Source: CAD feature listing. Evaluate the final solid. Frame: model axes, mm. A direction names the side the tool comes from. Give positions to 0.01 mm unless a question says otherwise; leave off trailing zeros. Order: outer loops, then holes, each group sorted by start corner. A loop starts at its lowest first (then second) coordinate and runs counter-clockwise, first axis right, second up. Notation, with made-up numbers: (60.25, 37.25) - (102.25, 37.25) arc R21 cw to (102.25, 46.25) - close; hole circle Ø9 at (27, 56). An arc over 180 degrees is marked (long way). Use CSV: the item, a comma, the result in double quotes.
```python
from build123d import *

# Parameters (mm, degrees)
F0_R     = 3.9142983579
F0_R_2   = 3.3882320549
F0_R_3   = 3.3768548991
F1_DEPTH = 2
F0_R_4   = 8.4535282778
F0_R_5   = 8.4613165319
F5_DEPTH = 6
F6_DEPTH = 6
F7_DEPTH = 6.096


# Not quite as in the source:
# - the program builds the solid bodies; features that only make, move or delete a surface that nothing else refers to are left out


with BuildPart() as f1:
    # F0 (on Top) → F1 (new body)
    with BuildSketch(Plane.XY):
        with BuildLine():
            Line((-5.016844254, 60.8599856496), (-5.016844254, 55.3855970502))
            Line((-5.016844254, 55.3855970502), (27.1643232554, 55.3855970502))
            Line((27.1643232554, 55.3855970502), (27.1643232554, 72.5930482149))
            ThreePointArc((27.1643232554, 72.5930482149), (15.3743446714, 74.0537278173), (9.8619121261, 84.5775231091))
            ThreePointArc((9.8619121261, 84.5775231091), (-38.0783668351, 114.5002429814), (-86.734496244, 85.7561899899))
            ThreePointArc((-86.734496244, 85.7561899899), (-89.789886214, 77.2334083533), (-97.5642204285, 72.5930482149))
            Line((-97.5642204285, 72.5930482149), (-97.5642204285, 55.3855970502))
            Line((-97.5642204285, 55.3855970502), (-82.5288370252, 55.3855970502))
            Line((-82.5288370252, 55.3855970502), (-62.9575885832, 55.3855970502))
            Line((-62.9575885832, 55.3855970502), (-62.9575885832, 60.8599856496))
            ThreePointArc((-62.9575885832, 60.8599856496), (-33.9872164186, 89.8303578142), (-5.016844254, 60.8599856496))
        make_face()
        with Locations((-86.9268402457, 61.0230416059)):
            Circle(F0_R, mode=Mode.SUBTRACT)
        with Locations((-72.1179321408, 60.8599856496)):
            Circle(F0_R, mode=Mode.SUBTRACT)
        with Locations((-68.8042789698, 85.551418364)):
            Circle(F0_R_2, mode=Mode.SUBTRACT)
        with Locations((4.3670018204, 60.8045533299)):
            Circle(F0_R, mode=Mode.SUBTRACT)
        with Locations((19.1759099253, 60.7153773308)):
            Circle(F0_R, mode=Mode.SUBTRACT)
        with Locations((-0.4634411598, 85.6597200036)):
            Circle(F0_R_3, mode=Mode.SUBTRACT)
        with Locations((-56.8258166313, 96.0706025362)):
            Circle(F0_R_3, mode=Mode.SUBTRACT)
        with Locations((-42.8707525134, 101.2179628015)):
            Circle(F0_R_3, mode=Mode.SUBTRACT)
        with Locations((-11.1492751166, 95.5843403935)):
            Circle(F0_R_3, mode=Mode.SUBTRACT)
        with Locations((-24.9121841043, 101.1035814881)):
            Circle(F0_R_3, mode=Mode.SUBTRACT)
    extrude(amount=F1_DEPTH)

    # F0 (on Top) → F5 (join)
    with BuildSketch(Plane.XY):
        with BuildLine():
            ThreePointArc((30.7714908133, 66.0106175583), (42.611434574, 81.0345848644), (36.6692617536, 99.2168411613))
            ThreePointArc((36.6692617536, 99.2168411613), (-37.7049289316, 128.8806796099), (-111.8238263521, 98.5845974088))
            ThreePointArc((-111.8238263521, 98.5845974088), (-116.4247817384, 79.7587957054), (-100.7084514224, 68.4196351703))
            Line((-100.7084514224, 68.4196351703), (-100.7084514224, 49.9112084508))
            Line((-100.7084514224, 49.9112084508), (-62.9575885832, 49.9112084508))
            Line((-62.9575885832, 49.9112084508), (-62.9575885832, 55.3855970502))
            Line((-62.9575885832, 55.3855970502), (-82.5288370252, 55.3855970502))
            Line((-82.5288370252, 55.3855970502), (-97.5642204285, 55.3855970502))
            Line((-97.5642204285, 55.3855970502), (-97.5642204285, 72.5930482149))
            ThreePointArc((-97.5642204285, 72.5930482149), (-89.789886214, 77.2334083533), (-86.734496244, 85.7561899899))
            ThreePointArc((-86.734496244, 85.7561899899), (-38.0783668351, 114.5002429814), (9.8619121261, 84.5775231091))
            ThreePointArc((9.8619121261, 84.5775231091), (15.3743446714, 74.0537278173), (27.1643232554, 72.5930482149))
            Line((27.1643232554, 72.5930482149), (27.1643232554, 55.3855970502))
            Line((27.1643232554, 55.3855970502), (-5.016844254, 55.3855970502))
            Line((-5.016844254, 55.3855970502), (-5.016844254, 49.9112084508))
            Line((-5.016844254, 49.9112084508), (30.7714908133, 49.9112084508))
            Line((30.7714908133, 49.9112084508), (30.7714908133, 66.0106175583))
        make_face()
        with Locations((-100.1490219674, 85.7561899899)):
            Circle(F0_R_4, mode=Mode.SUBTRACT)
        with Locations((22.6636270451, 84.5775231091)):
            Circle(F0_R_5, mode=Mode.SUBTRACT)
    extrude(amount=F5_DEPTH)

    # F0 (on Top) → F6 (join)
    with BuildSketch(Plane.XY):
        with BuildLine():
            ThreePointArc((30.7714908133, 66.0106175583), (42.611434574, 81.0345848644), (36.6692617536, 99.2168411613))
            ThreePointArc((36.6692617536, 99.2168411613), (-37.7049289316, 128.8806796099), (-111.8238263521, 98.5845974088))
            ThreePointArc((-111.8238263521, 98.5845974088), (-116.4247817384, 79.7587957054), (-100.7084514224, 68.4196351703))
            Line((-100.7084514224, 68.4196351703), (-100.7084514224, 49.9112084508))
            Line((-100.7084514224, 49.9112084508), (-62.9575885832, 49.9112084508))
            Line((-62.9575885832, 49.9112084508), (-62.9575885832, 55.3855970502))
            Line((-62.9575885832, 55.3855970502), (-82.5288370252, 55.3855970502))
            Line((-82.5288370252, 55.3855970502), (-97.5642204285, 55.3855970502))
            Line((-97.5642204285, 55.3855970502), (-97.5642204285, 72.5930482149))
            ThreePointArc((-97.5642204285, 72.5930482149), (-89.789886214, 77.2334083533), (-86.734496244, 85.7561899899))
            ThreePointArc((-86.734496244, 85.7561899899), (-38.0783668351, 114.5002429814), (9.8619121261, 84.5775231091))
            ThreePointArc((9.8619121261, 84.5775231091), (15.3743446714, 74.0537278173), (27.1643232554, 72.5930482149))
            Line((27.1643232554, 72.5930482149), (27.1643232554, 55.3855970502))
            Line((27.1643232554, 55.3855970502), (-5.016844254, 55.3855970502))
            Line((-5.016844254, 55.3855970502), (-5.016844254, 49.9112084508))
            Line((-5.016844254, 49.9112084508), (30.7714908133, 49.9112084508))
            Line((30.7714908133, 49.9112084508), (30.7714908133, 66.0106175583))
        make_face()
        with Locations((-100.1490219674, 85.7561899899)):
            Circle(F0_R_4, mode=Mode.SUBTRACT)
        with Locations((22.6636270451, 84.5775231091)):
            Circle(F0_R_5, mode=Mode.SUBTRACT)
    extrude(amount=F6_DEPTH)

    # F0 (on Top) → F7 (join)
    with BuildSketch(Plane.XY):
        with BuildLine():
            ThreePointArc((30.7714908133, 66.0106175583), (42.611434574, 81.0345848644), (36.6692617536, 99.2168411613))
            ThreePointArc((36.6692617536, 99.2168411613), (-37.7049289316, 128.8806796099), (-111.8238263521, 98.5845974088))
            ThreePointArc((-111.8238263521, 98.5845974088), (-116.4247817384, 79.7587957054), (-100.7084514224, 68.4196351703))
            Line((-100.7084514224, 68.4196351703), (-100.7084514224, 49.9112084508))
            Line((-100.7084514224, 49.9112084508), (-62.9575885832, 49.9112084508))
            Line((-62.9575885832, 49.9112084508), (-62.9575885832, 55.3855970502))
            Line((-62.9575885832, 55.3855970502), (-82.5288370252, 55.3855970502))
            Line((-82.5288370252, 55.3855970502), (-97.5642204285, 55.3855970502))
            Line((-97.5642204285, 55.3855970502), (-97.5642204285, 72.5930482149))
            ThreePointArc((-97.5642204285, 72.5930482149), (-89.789886214, 77.2334083533), (-86.734496244, 85.7561899899))
            ThreePointArc((-86.734496244, 85.7561899899), (-38.0783668351, 114.5002429814), (9.8619121261, 84.5775231091))
            ThreePointArc((9.8619121261, 84.5775231091), (15.3743446714, 74.0537278173), (27.1643232554, 72.5930482149))
            Line((27.1643232554, 72.5930482149), (27.1643232554, 55.3855970502))
            Line((27.1643232554, 55.3855970502), (-5.016844254, 55.3855970502))
            Line((-5.016844254, 55.3855970502), (-5.016844254, 49.9112084508))
            Line((-5.016844254, 49.9112084508), (30.7714908133, 49.9112084508))
            Line((30.7714908133, 49.9112084508), (30.7714908133, 66.0106175583))
        make_face()
        with Locations((-100.1490219674, 85.7561899899)):
            Circle(F0_R_4, mode=Mode.SUBTRACT)
        with Locations((22.6636270451, 84.5775231091)):
            Circle(F0_R_5, mode=Mode.SUBTRACT)
    extrude(amount=F7_DEPTH)


solid = f1.part
```
Item 1: Section A-A on z = 5. Return the cut outline in (x, y).
Filled in:
outline,"(-111.82, 98.58) arc R17.35 ccw to (-100.71, 68.42) - (-100.71, 49.91) - (-62.96, 49.91) - (-62.96, 55.39) - (-97.56, 55.39) - (-97.56, 72.59) arc R13.41 ccw to (-86.73, 85.76) arc R54.43 cw to (9.86, 84.58) arc R12.8 ccw to (27.16, 72.59) - (27.16, 55.39) - (-5.02, 55.39) - (-5.02, 49.91) - (30.77, 49.91) - (30.77, 66.01) arc R20.26 ccw to (36.67, 99.22) arc R106.93 ccw to start; hole circle Ø16.91 at (-100.15, 85.76); hole circle Ø16.92 at (22.66, 84.58)"
Item 2: Set-up query: faces 1 (the flat face through (-97.564, 64, 4)), 2 (the flat face through (30.771, 58, 3)), 3 (the flat face through (-62.958, 54, 2)), 4 (the cylindrical face through (-66.983, 88.408, 0.986)). Return all of +Z, -Z, +X, -X, +Y, -Y with unobstructed straight access to the full face (end or side cutting, diameter ignored); none if empty.
Filled in:
face 1,"+Z"
face 2,"+Z, -Z, +X, -Y"
face 3,"+Z, -Z, -Y"
face 4,"+Z, -Z"
Item 3: Mould query, pull axis Y, two halves, no side actions, for faces 5 (the cylindrical face through (-23.35, 98.11, 0.99)), 6 (the flat face through (-38, 90, 0)), 7 (the cylindrical face through (42.56, 80.76, 3.01)), 8 (the cylindrical face through (-87.436, 64.904, 0.986)). Classes: released by +Y, released by -Y, zero draft, split by the parting line, or undercut.
Filled in:
face 5,"undercut"
face 6,"zero draft"
face 7,"split by the parting line"
face 8,"undercut"
Item 4: Section B-B on x = -26. Return the cut outline in (y, z).
Filled in:
outline,"(88.71, 0) - (97.91, 0) - (97.91, 2) - (88.71, 2) - close; (104.3, 0) - (128.29, 0) - (128.29, 6.1) - (112.99, 6.1) - (112.99, 2) - (104.3, 2) - close"
Item 5: Section D-D on y = 108.5. Return the cut outline in (x, z).
Filled in:
outline,"(-100.05, 0) - (25.55, 0) - (25.55, 6.1) - (-13.89, 6.1) - (-13.89, 2) - (-63.59, 2) - (-63.59, 6.1) - (-100.05, 6.1) - close"
Item 6: Material intervals for line 1 (X direction, y = 78.5, z = 4.5); line 2 (X direction, y = 86.5, z = 0.75); line 3 (X direction, y = 56.5, z = 0.75), sorted ascending. Write a range as from..to.
Filled in:
line 1,"x = -115.9..-104.49, -95.81..-88.87, 11.4..16.78, 28.55..41.99"
line 2,"x = -117.48..-108.57, -91.73..-72.06, -65.55..-47.47, -20.5..-3.73, 2.81..14.42, 30.9..42.83"
line 3,"x = -100.71..-62.96, -5.02..30.77"
Item 7: First-contact query: pin 1 (8 mm diameter, centred on x = -80, y = 82, fed in from +Z); pin 2 (2 mm diameter, centred on y = 62, z = 3.5, fed in from -X); pin 3 (1.5 mm diameter, centred on y = 81, z = 4.5, fed in from -X). Flat tips, straight axial feed; report the tip coordinate or a pass-through.
Filled in:
pin 1,"stops at z = 2"
pin 2,"stops at x = -100.71"
pin 3,"stops at x = -117.03"
Item 8: Section C-C on x = -78. Return the cut outline in (y, z), then the cut area to 3 significant figures.
Filled in:
outline,"(49.91, 0) - (120.81, 0) - (120.81, 6.1) - (97.78, 6.1) - (97.78, 2) - (55.39, 2) - (55.39, 6.1) - (49.91, 6.1) - close"
area,"259 mm2"
